Input: part model. Units: mm. Frame: model coordinates. Face numbers are marked on the shaded views. A direction names the side the tool comes from. Coordinates: 2 decimals unless noted, no trailing zeros. Write each loop counter-clockwise with the first axis right and the second up, starting at its lowest first coordinate (ties: lowest second). Pieces come first, ordered by that corner, then holes.
1) Section query C-C (y = 15.5). Output: boundary loops of the cut face in (x, z), then the cut area to 3 significant figures.
2) Section query A-A (x = 43). Output: boundary loops of the cut face in (y, z), then the cut area to 3 significant figures.
3) Pin query (flat end, axial travel): pin 1 Ø6 at (x, y) = (54, 26.5) entering from +Z; pin 2 Ø10 at (x, z) = (43, -21) entering from +Y; pin 3 Ø6 at (x, z) = (37, -35.5) entering from -Y; pin 4 Ø3 at (x, z) = (31, -18.5) entering from +Y. Return the tip coordinate at first contact, or that it passes through.
4) Set-up query: the marked faces 1 and 2. Return all of +Z, -Z, +X, -X, +Y, -Y with unobstructed straight access to the full face (end or side cutting, diameter ignored); none if empty.
5) Line query: L1, parallel to Y at x = 36, z = -2; L2, parallel to Y at x = 61.5, z = -8.5; L3, parallel to X at y = 29, z = -20. Output: solid intervals per line, ascending.
6) Section query B-B (z = -10.5). Output: boundary loops of the cut face in (x, y), then the cut area to 3 significant figures.
7) Section query D-D (x = 35). Output: boundary loops of the cut face in (y, z).
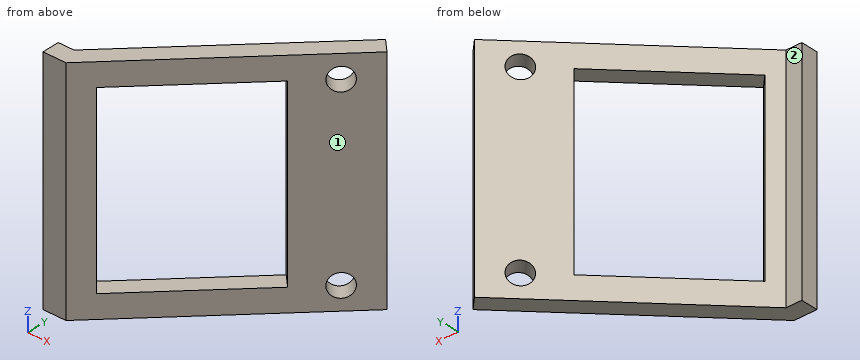
from build123d import *

# Parameters (mm, degrees)
PAD001_DEPTH    = 40
SKETCH002_R     = 2
POCKET_DEPTH    = 5
SKETCH003_W     = 14.874642
SKETCH003_H     = 51.167498
SKETCH003_W_2   = 25
SKETCH003_H_2   = 32
POCKET001_DEPTH = 5


with BuildPart() as part:
    # Sketch001 → Pad001 (new body)
    with BuildSketch(Plane.XY):
        Polygon((33.191021, 0), (65.010826, 31.819805), (62.889506, 33.941125), (31.948381, 3), (29.191021, 3), (29.191021, 0), align=None)
    extrude(amount=-PAD001_DEPTH)

    # Sketch002 → Pocket (cut)
    with BuildSketch(Plane(origin=(16.595511, -16.595511, 0), x_dir=(0.707107, 0.707107, 0), z_dir=(0.707107, -0.707107, 0))):
        with Locations((59.469596, -36)):
            Circle(SKETCH002_R)
        with Locations((59.469596, -4)):
            Circle(SKETCH002_R)
    extrude(amount=-POCKET_DEPTH, mode=Mode.SUBTRACT)

    # Sketch003 → Pocket001 (cut)
    with BuildSketch(Plane(origin=(16.595511, -16.595511, 0), x_dir=(0.707107, 0.707107, 0), z_dir=(0.707107, -0.707107, 0))):
        with Locations((72.906917, -16.654673)):
            Rectangle(SKETCH003_W, SKETCH003_H)
        with Locations((39.969596, -20)):
            Rectangle(SKETCH003_W_2, SKETCH003_H_2)
    extrude(amount=-POCKET001_DEPTH, mode=Mode.SUBTRACT)


solid = part.part
Answer:
1. outline: (44.45, -40) - (48.69, -40) - (48.69, -36) - (44.45, -36) - close; (44.45, -4) - (48.69, -4) - (48.69, 0) - (44.45, 0) - close
1. area: 33.9 mm2
2. outline: (9.81, -40) - (14.05, -40) - (14.05, -36) - (9.81, -36) - close; (9.81, -4) - (14.05, -4) - (14.05, 0) - (9.81, 0) - close
2. area: 33.9 mm2
3. pin 1: stops at z = 0
3. pin 2: passes through
3. pin 3: stops at y = 0.81
3. pin 4: stops at y = 3.55
4. face 1: +Z, -Z, +X, -Y
4. face 2: +Z, -Z, -X, +Y
5. L1: y = 2.81 to 7.05
5. L2: y = 28.31 to 31.09
5. L3: x = 57.95 to 62.19
6. outline: (29.19, 0) - (33.19, 0) - (36.02, 2.83) - (33.9, 4.95) - (31.95, 3) - (29.19, 3) - close; (51.58, 22.63) - (53.7, 20.51) - (62.89, 29.7) - (60.77, 31.82) - close
6. area: 59.3 mm2
7. outline: (1.81, -40) - (6.05, -40) - (6.05, -36) - (3.85, -36) - (3.85, -4) - (6.05, -4) - (6.05, 0) - (1.81, 0) - close
